Drawing for the job (mm, zero at the part's lowest x, y, z). A direction names the side the tool comes from. Coordinates: 2 decimals unless noted, no trailing zeros. Order: outer loops, then holes, each group sorted by start corner. A loop starts at its lowest first (then second) coordinate and runs counter-clockwise, first axis right, second up.
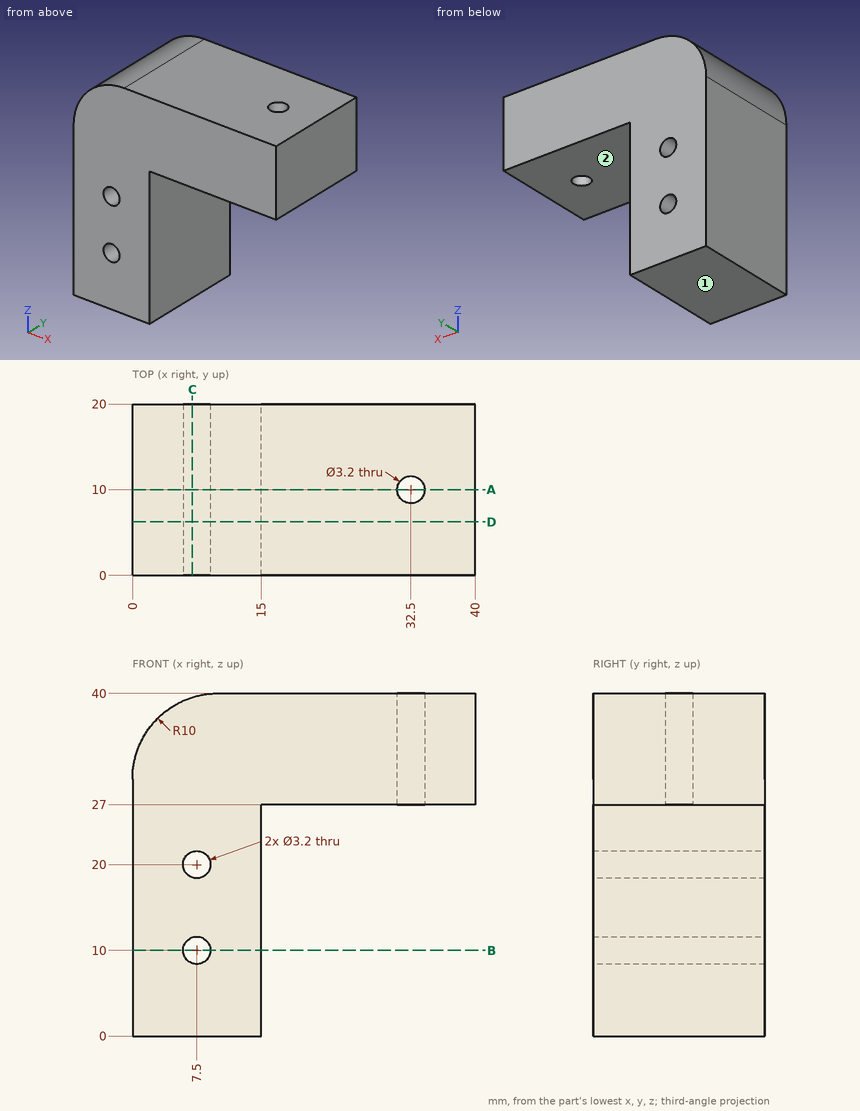
(1) Probe line 1 (X direction, y = 11, z = 20); line 2 (X direction, y = 7, z = 22); line 3 (Z direction, x = 26, y = 11.75). List the from-to ranges inside material, lowest first.
(2) Slice it at A-A, the plane y = 10. Give the cut face in (x, z).
(3) Slice it at D-D, the plane y = 6.25. Give the cut face in (x, z).
(4) Drop flat-ended pins along their axis: pin 1 (3 mm diameter, centred on x = 30.5, y = 11.5, fed in from -Z); pin 2 (6 mm diameter, centred on y = 13.5, z = 22, fed in from +X). Give the stop position or say it passes through.
(5) Slice it at C-C, the plane x = 7. Give the cut face in (y, z), then the cut area to 3 significant figures.
(6) Tool access for the marked faces 1 and 2: list every direction of +Z, -Z, +X, -X, +Y, -Y with a clear straight run to the whole face (end or side of a thin tool).
(7) Slice it at B-B, the plane z = 10. Give the cut face in (x, y).
Here are the results:
1. line 1: x = 0 to 5.9, 9.1 to 15
1. line 2: x = 0 to 15
1. line 3: z = 27 to 40
2. outline: (0, 0) - (15, 0) - (15, 27) - (30.9, 27) - (30.9, 40) - (10, 40) arc R10 ccw to (0, 30) - close; (34.1, 27) - (40, 27) - (40, 40) - (34.1, 40) - close; hole circle Ø3.2 at (7.5, 10); hole circle Ø3.2 at (7.5, 20)
3. outline: (0, 0) - (15, 0) - (15, 27) - (40, 27) - (40, 40) - (10, 40) arc R10 ccw to (0, 30) - close; hole circle Ø3.2 at (7.5, 10); hole circle Ø3.2 at (7.5, 20)
4. pin 1: stops at z = 27
4. pin 2: stops at x = 15
5. outline: (0, 0) - (20, 0) - (20, 8.48) - (0, 8.48) - close; (0, 11.52) - (20, 11.52) - (20, 18.48) - (0, 18.48) - close; (0, 21.52) - (20, 21.52) - (20, 39.54) - (0, 39.54) - close
5. area: 669 mm2
6. face 1: -Z, +X, -X, +Y, -Y
6. face 2: -Z, +X, +Y, -Y
7. outline: (0, 0) - (5.9, 0) - (5.9, 20) - (0, 20) - close; (9.1, 0) - (15, 0) - (15, 20) - (9.1, 20) - close
